```python
from build123d import *

# Parameters (mm, degrees)
SKETCH_1_R         = 8.75
EXTRUDE_1_DEPTH    = 5.5
DOME_1_FACE_RADIUS = 8.75
DOME_1_HEIGHT      = 10


# Read off the part's stored shape, not the designer's step: 抽壳1
with BuildPart() as part:
    # 草图1 → 凸台-拉伸1 (new body)
    with BuildSketch(Plane(origin=(0, 0, 0), x_dir=(1, 0, 0), z_dir=(0, 1, 0))):
        with Locations(Location((0, 0, 0), (0, 0, 270))):
            Circle(SKETCH_1_R)
    extrude(amount=EXTRUDE_1_DEPTH)

    # 圆顶1: a dome of height H over a round flat face of radius A is a cap of a sphere of radius (A * A + H * H) / (2 * H)
    dome_1_r = (DOME_1_FACE_RADIUS * DOME_1_FACE_RADIUS + DOME_1_HEIGHT * DOME_1_HEIGHT) / (2 * DOME_1_HEIGHT)
    dome_1_base = Plane((0, 5.5, 0), z_dir=(0, 1, 0))
    with Locations(dome_1_base.offset(DOME_1_HEIGHT - dome_1_r)):
        dome_1_ball = Sphere(dome_1_r, mode=Mode.PRIVATE)
    add(split(dome_1_ball, bisect_by=dome_1_base, keep=Keep.TOP, mode=Mode.PRIVATE))

    # 抽壳1 outline → 抽壳1 (revolve, cut)
    with BuildSketch(Plane.XY):
        with BuildLine():
            Line((0, 13.5), (0, 0))
            Line((0, 0), (6.75, 0))
            Line((6.75, 0), (6.75, 5.641927904))
            ThreePointArc((6.75, 5.641927904), (5.179570375, 11.12107063), (0, 13.5))
        make_face()
    revolve(axis=Axis((0, 0, 0), (0, 1, 0)), mode=Mode.SUBTRACT)


solid = part.part
```
The model under review builds one solid part; all positions refer to its coordinate system, in mm. Round coordinates to 2 decimals unless told otherwise and drop trailing zeros. Loops run counter-clockwise (first coordinate to the right, second up) from the corner with the lowest first, then second, coordinate; pieces in that order, holes last. Notation, with made-up numbers: M 82,3.5 L 100,3.5 A24 cw 100,36.5 Z; hole C 59,13 d1. An arc over 180 degrees is marked long. Answer as a JSON object with one key per item and string values.
(1) Take a section at C-C on y = 2.75. Give the boundary of the cut face in (x, z), and give its area (3 significant figures).
Resolved:
{"outline": "C 0,0 d17.5; hole C 0,0 d13.5", "area": "97.4 mm²"}
(2) Take a section at A-A on x = 0. Give the boundary of the cut face in (y, z), and give its area (3 significant figures).
Resolved:
{"outline": "M 0,-8.75 L 5.5,-8.75 A8.83 ccw long 5.5,8.75 L 0,8.75 L 0,6.75 L 5.64,6.75 A6.83 cw long 5.64,-6.75 L 0,-6.75 Z", "area": "75.9 mm²"}
(3) Take a section at B-B on z = 0. Give the boundary of the cut face in (x, y).
Resolved:
{"outline": "M -8.75,0 L -6.75,0 L -6.75,5.64 A6.83 cw long 6.75,5.64 L 6.75,0 L 8.75,0 L 8.75,5.5 A8.83 ccw long -8.75,5.5 Z"}
(4) Draft analysis for pull direction Z (two halves, no side actions). For faces 1 (the cylindrical face through (-5.324, 2.712, -6.944)), 2 (the cylindrical face through (-1.46, 2.86, 6.59)), 3 (the flat face through (-6.4, 0, 2.6)), state which applies: released by +Z, released by -Z, zero draft, split by the parting line, or undercut.
Resolved:
{"face 1": "split by the parting line", "face 2": "undercut", "face 3": "zero draft"}
(5) Take a section at D-D on x = -6.25. Give the boundary of the cut face in (y, z), and give its area (3 significant figures).
Resolved:
{"outline": "M 0,-6.12 L 5.5,-6.12 A6.23 ccw long 5.5,6.12 L 0,6.12 L 0,2.55 L 5.64,2.55 A2.75 cw long 5.64,-2.55 L 0,-2.55 Z", "area": "96.8 mm²"}
(6) To check wall thickness, follow line 1 along X through (y, z) = (1.8, 0); line 2 along Z through (x, y) = (0, 11); line 3 along Z through (x, y) = (-2.5, 10). State the ranges of each line that lie inside material, in increasing order.
Resolved:
{"line 1": "-8.75 to -6.75, 6.75 to 8.75", "line 2": "-7.69 to -5.28, 5.28 to 7.69", "line 3": "-7.79 to -5.41, 5.41 to 7.79"}
(7) Clearance check with flat-ended pins moving along their axes: P1, Ø1.5, axis at x = 6.5, y = 10.5, coming from the +Z side; P2, Ø4, axis at y = 4.5, z = 5, coming from the -X side; P3, Ø3, axis at x = -3, y = 11.5, coming from the +Z side. State where each tip first meets the part, or that it passes through.
Resolved:
{"P1": "z = 5.64", "P2": "x = -8.22", "P3": "z = 7.77"}
